Here's how the part is built. I have some questions about the finished solid (model axes, mm). A direction names the side the tool comes from. Round coordinates to 2 decimals unless told otherwise and drop trailing zeros. Order: outer loops, then holes, each group sorted by start corner. A loop starts at its lowest first (then second) coordinate and runs counter-clockwise, first axis right, second up. Notation, with made-up numbers: (64.5, 45) -> (94.5, 45) arc R20 ccw to (94.5, 83) -> close; hole circle Ø9 at (50.25, 83.5). An arc over 180 degrees is marked (long way). Answer in a Markdown table with one row per item.
```python
from build123d import *

# Parameters (mm, degrees)
F1_DEPTH = 8
F3_DEPTH = 2
F4_R     = 4
F5_DEPTH = 8
F7_DEPTH = 2


with BuildPart() as f1:
    # F0 (on Top) → F1 (new body)
    with BuildSketch(Plane.XY):
        with BuildLine():
            Line((-102, -360), (0, -360))
            ThreePointArc((0, -360), (360, 0), (0, 360))
            Line((0, 360), (-102, 360))
            Line((-102, 360), (-202, 360))
            Line((-202, 360), (-202, -360))
            Line((-202, -360), (-102, -360))
        make_face()
    extrude(amount=F1_DEPTH)

    # F2 (on face) → F3 (cut)
    with BuildSketch(Plane(origin=(0, 0, 0), x_dir=(1, 0, 0), z_dir=(0, 0, -1))):
        with BuildLine():
            ThreePointArc((0, 350), (350, 0), (0, -350))
            Line((0, -350), (-202, -350))
            Line((-202, -350), (-202, -352))
            Line((-202, -352), (0, -352))
            ThreePointArc((0, -352), (352, 0), (0, 352))
            Line((0, 352), (-202, 352))
            Line((-202, 352), (-202, 350))
            Line((-202, 350), (0, 350))
        make_face()
    extrude(amount=-F3_DEPTH, mode=Mode.SUBTRACT)

    # F4 (on face) → F5 (cut, through all)
    with BuildSketch(Plane.XY.offset(8)):
        with Locations((-32, 47)):
            Circle(F4_R)
    extrude(amount=-F5_DEPTH, mode=Mode.SUBTRACT)

    # F6 (on face) → F7 (cut)
    with BuildSketch(Plane(origin=(0, 0, 0), x_dir=(1, 0, 0), z_dir=(0, 0, -1))):
        with BuildLine():
            Line((-202, -149), (-102, -149))
            ThreePointArc((-102, -149), (-29.875108278, -119.1248916401), (0, -46.9999998841))
            ThreePointArc((0, -46.9999998841), (-29.8751083599, 25.124891722), (-102, 55))
            Line((-102, 55), (-202, 55))
            Line((-202, 55), (-202, -149))
        make_face()
    extrude(amount=-F7_DEPTH, mode=Mode.SUBTRACT)


solid = f1.part
```
1. Suppose I cut it at D-D on y = 137. Write out the boundary of the cut face in (x, z), then the cut area to 3 significant figures.
Numbers:
| item | result |
|---|---|
| outline | (-202, 2) -> (-54, 2) -> (-54, 0) -> (322.07, 0) -> (322.07, 2) -> (324.25, 2) -> (324.25, 0) -> (332.91, 0) -> (332.91, 8) -> (-202, 8) -> close |
| area | 3,980 mm2 |
2. Suppose I cut it at C-C on y = 0. Write out the boundary of the cut face in (x, z).
Numbers:
| item | result |
|---|---|
| outline | (-202, 2) -> (-11.47, 2) -> (-11.47, 0) -> (350, 0) -> (350, 2) -> (352, 2) -> (352, 0) -> (360, 0) -> (360, 8) -> (-202, 8) -> close |
3. Suppose I cut it at A-A on z = 4.25. Write out the boundary of the cut face in (x, y), then the cut area to 3 significant figures.
Numbers:
| item | result |
|---|---|
| outline | (-202, -360) -> (0, -360) arc R360 ccw to (0, 360) -> (-202, 360) -> close; hole circle Ø8 at (-32, 47) |
| area | 349,000 mm2 |
4. For pin 1 Ø13 at (x, y) = (-32, 47) entering from -Z; pin 2 Ø3 at (y, z) = (-189.5, 2) entering from +X, each with a flat end and sliding along its axis, tell me the tip position at first contact or that it passes through.
Numbers:
| item | result |
|---|---|
| pin 1 | stops at z = 2 |
| pin 2 | stops at x = 307.01 |
5. We'd pull the mould along X, two halves only. Please class faces 4 (the face through (349.915, -7.696, 0.986)), 5 (the face through (359.913, -7.916, 3.944)), 6 (the face through (348, 55, 0)): released by +X, released by -X, zero draft, split by the parting line, or undercut.
Numbers:
| item | result |
|---|---|
| face 4 | undercut |
| face 5 | released by +X |
| face 6 | zero draft |
6. For faces 1 (the face through (-102, 46, 2)), 2 (the face through (351.915, 7.74, 0.986)), 3 (the face through (70, 5, 0)), which set-ups out of +Z, -Z, +X, -X, +Y, -Y let a thin tool reach every point of the face, with its end or its side?
Numbers:
| item | result |
|---|---|
| face 1 | -Z, -X |
| face 2 | -Z |
| face 3 | -Z, +X, -X, +Y, -Y |
7. Please list where these lines run through material, in increasing order: line 1 along Y through (x, z) = (-32, 4.2); line 2 along Z through (x, y) = (-72.5, -43); line 3 along X through (y, z) = (62.5, 1.75).
Numbers:
| item | result |
|---|---|
| line 1 | y = -360 to 43, 51 to 360 |
| line 2 | z = 2 to 8 |
| line 3 | x = -1.18 to 344.37, 346.41 to 354.53 |
8. Suppose I cut it at B-B on x = -111.5. Write out the boundary of the cut face in (y, z).
Numbers:
| item | result |
|---|---|
| outline | (-360, 0) -> (-352, 0) -> (-352, 2) -> (-350, 2) -> (-350, 0) -> (-55, 0) -> (-55, 2) -> (149, 2) -> (149, 0) -> (350, 0) -> (350, 2) -> (352, 2) -> (352, 0) -> (360, 0) -> (360, 8) -> (-360, 8) -> close |
